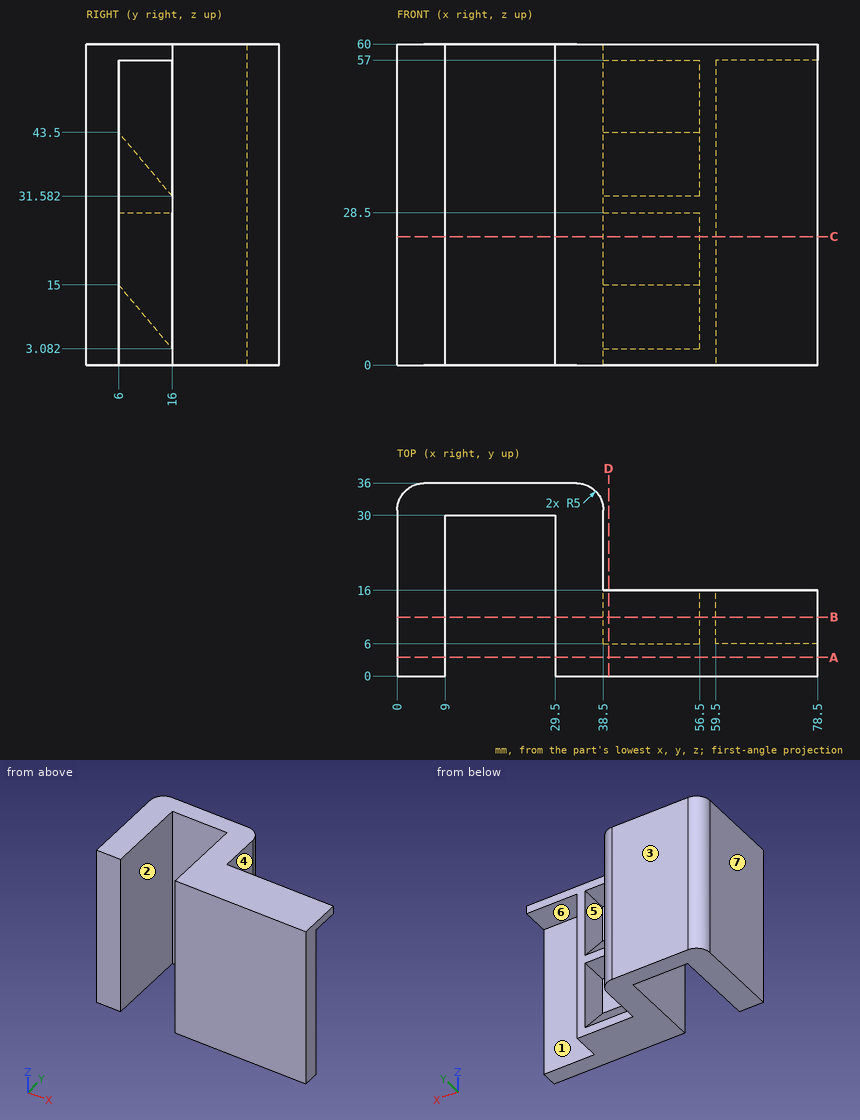
Geometry: see drawing. Coordinates: mm, zero at the bounding-box minimum. A direction names the side the tool comes from. Coordinates: 2 decimals unless noted, no trailing zeros. Loops run counter-clockwise (first coordinate to the right, second up) from the corner with the lowest first, then second, coordinate; pieces in that order, holes last. Notation, with made-up numbers: (60.5, 40) - (73.5, 40) arc R9 cw to (73.5, 49) - close; hole circle Ø1 at (84, 78). An arc over 180 degrees is marked (long way). Put each result on its own line as item: value. Start each with the question number.
Q1. Cut plane D-D, the plane x = 39.5. Return loops of the section in (y, z), and give its area (3 significant figures).
Q2. Set-up query: the marked faces 1, 2, 3 and 4. Return all of +Z, -Z, +X, -X, +Y, -Y with unobstructed straight access to the full face (end or side cutting, diameter ignored); none if empty.
Q3. Cut plane A-A, the plane y = 3.5. Return loops of the section in (x, z).
Q4. Cut plane C-C, the plane z = 24. Return loops of the section in (x, y).
Q5. Pin query (flat end, axial travel): pin 1 Ø21 at (x, z) = (71, 34) entering from +Y; pin 2 Ø3 at (x, y) = (69.5, 11) entering from -Z; pin 3 Ø5 at (y, z) = (10.5, 34) entering from +X. Return the tip coordinate at first contact, or that it passes through.
Q6. Cut plane B-B, the plane y = 11. Return loops of the section in (x, z).
Q7. Pull-direction query (Z, two-part tool) for the marked faces 5, 6 and 7; classes: released by +Z, released by -Z, zero draft, split by the parting line, or undercut.
Q8. Line query: line 1 (X direction, y = 14.5, z = 5); line 2 (X direction, y = 7, z = 29); line 3 (X direction, y = 20, z = 32). Output: solid intervals per line, ascending.
Filled sheet:
1. outline: (0, 0) - (16, 0) - (16, 3.08) - (6, 15) - (6, 28.5) - (16, 28.5) - (16, 31.58) - (6, 43.5) - (6, 57) - (16, 57) - (16, 60) - (0, 60) - close
1. area: 571 mm²
2. face 1: -Z, +X, +Y
2. face 2: +Z, -Z, -Y
2. face 3: +Z, -Z, +X, -X, +Y
2. face 4: +Y
3. outline: (0, 0) - (9, 0) - (9, 60) - (0, 60) - close; (29.5, 0) - (78.5, 0) - (78.5, 60) - (29.5, 60) - close
4. outline: (0, 0) - (9, 0) - (9, 30) - (29.5, 30) - (29.5, 0) - (78.5, 0) - (78.5, 6) - (59.5, 6) - (59.5, 16) - (56.5, 16) - (56.5, 6) - (38.5, 6) - (38.5, 31) arc R5 ccw to (33.5, 36) - (5, 36) arc R5 ccw to (0, 31) - close
5. pin 1: y = 6
5. pin 2: z = 57
5. pin 3: x = 59.5
6. outline: (0, 0) - (9, 0) - (9, 60) - (0, 60) - close; (29.5, 0) - (59.5, 0) - (59.5, 57) - (78.5, 57) - (78.5, 60) - (29.5, 60) - close; hole (38.5, 9.04) - (56.5, 9.04) - (56.5, 28.5) - (38.5, 28.5) - close; hole (38.5, 37.54) - (56.5, 37.54) - (56.5, 57) - (38.5, 57) - close
7. face 5: undercut
7. face 6: released by -Z
7. face 7: zero draft
8. line 1: 0 to 9, 29.5 to 38.5, 56.5 to 59.5
8. line 2: 0 to 9, 29.5 to 59.5
8. line 3: 0 to 9, 29.5 to 38.5
